Read the model definition and answer for the solid it produces. Units are mm, in the model's axes. Face numbers are marked on the shaded views. A direction names the side the tool comes from. Round coordinates to 2 decimals unless told otherwise and drop trailing zeros. Write each loop counter-clockwise with the first axis right and the second up, starting at its lowest first coordinate (ties: lowest second). Pieces come first, ordered by that corner, then holes. Notation, with made-up numbers: (8, 43) -> (13, 43) arc R6 cw to (13, 51) -> close; hole circle Ø8 at (30.5, 72). An arc over 180 degrees is marked (long way). Return JSON: item names as keys, results as strings. Group by question number.
(1) Given pin 1 (5.5 mm diameter, centred on x = 39, y = 5, fed in from -Z); pin 2 (8 mm diameter, centred on x = 39, y = 5, fed in from +Z); pin 3 (1.4 mm diameter, centred on x = 43.5, z = -7.5, fed in from -Y); pin 4 (2 mm diameter, centred on x = 26, y = -9.2, fed in from -Z), each flat-ended and moving along its own axis, determine where each tip first touches the part or whether it passes through.
(2) A cutting plane is placed at B-B on z = -11.25. Give the vertices of the cut face in (x, y).
(3) A cutting plane is placed at C-C on z = -8. Give the vertices of the cut face in (x, y), then the cut area to 3 significant figures.
(4) For the marked faces 4, 5 and 6, determine the directions among +Z, -Z, +X, -X, +Y, -Y from which every point of the face is accessible in a straight line to the end or side of a thin tool.
(5) A cutting plane is placed at A-A on x = 26. Give the vertices of the cut face in (y, z).
(6) Straight lines are drawn through the part: line 1 (X direction, y = 5, z = -11.05); line 2 (X direction, y = 6.25, z = -4.75); line 3 (Z direction, x = 29, y = 1.75). For each, find the intervals that lie inside material, in ascending order.
(7) A cutting plane is placed at D-D on x = 38.5. Give the vertices of the cut face in (y, z), then the cut area to 3 significant figures.
(8) The mould has two halves that part along X. Classify the marked faces 1, 2 and 3: released by +X, released by -X, zero draft, split by the parting line, or undercut.
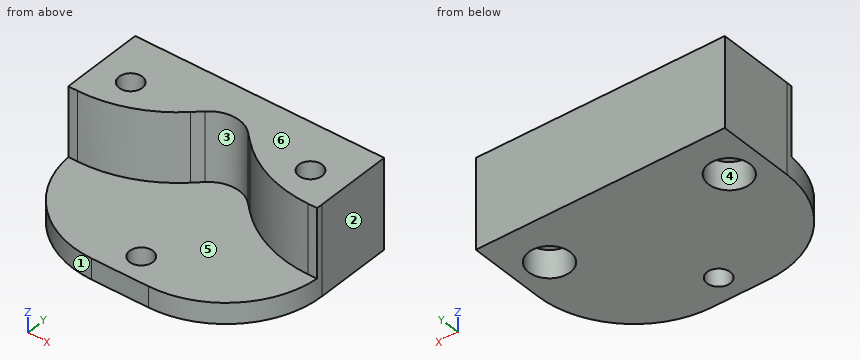
```python
from build123d import *

# Parameters (mm, degrees)
BOX001_W        = 36
BOX001_H        = 25
BOX001_DEPTH    = 13
SKETCH_R        = 1.68
POCKET005_DEPTH = 13.001
SKETCH014_W     = 13
SKETCH014_H     = 10
POCKET006_DEPTH = 36.001
SKETCH015_R     = 3
POCKET007_DEPTH = 4
POCKET008_DEPTH = 10
FILLET_R        = 18
FILLET001_R     = 4.5
FILLET002_R     = 13.9


with BuildPart() as part:
    # Box001 → Box001 (new body)
    with BuildSketch(Plane(origin=(8, -13, -13), x_dir=(1, 0, 0), z_dir=(0, 0, 1))):
        with Locations((18, 12.5)):
            Rectangle(BOX001_W, BOX001_H)
    extrude(amount=BOX001_DEPTH)

    # Sketch → Pocket005 (cut, through all)
    with BuildSketch(Plane(origin=(8, -13, -13), x_dir=(1, 0, 0), z_dir=(0, 0, -1))):
        with Locations((31, -18)):
            Circle(SKETCH_R)
        with Locations((5, -18)):
            Circle(SKETCH_R)
        with Locations((18, -3.8)):
            Circle(SKETCH_R)
    extrude(amount=-POCKET005_DEPTH, mode=Mode.SUBTRACT)

    # Sketch014 → Pocket006 (cut, through all)
    with BuildSketch(Plane(origin=(8, -13, -13), x_dir=(0, -1, 0), z_dir=(-1, 0, 0))):
        with Locations((-6.5, 8)):
            Rectangle(SKETCH014_W, SKETCH014_H)
    extrude(amount=-POCKET006_DEPTH, mode=Mode.SUBTRACT)

    # Sketch015 → Pocket007 (cut)
    with BuildSketch(Plane(origin=(8, -13, -13), x_dir=(1, 0, 0), z_dir=(0, 0, -1))):
        with Locations((5, -18)):
            Circle(SKETCH015_R)
        with Locations((31, -18)):
            Circle(SKETCH015_R)
    extrude(amount=-POCKET007_DEPTH, mode=Mode.SUBTRACT)

    # Sketch016 → Pocket008 (cut)
    with BuildSketch(Plane(origin=(8, -13, 0), x_dir=(1, 0, 0), z_dir=(0, 0, 1))):
        Polygon((8.5, 13), (18, 22), (27.5, 13), align=None)
    extrude(amount=-POCKET008_DEPTH, mode=Mode.SUBTRACT)

    # Fillet
    fillet_edges = [part.edges().sort_by_distance(p)[0] for p in [
        (16.5, 0, -5),
        (35.5, 0, -5),
    ]]
    fillet(fillet_edges, radius=FILLET_R)

    # Fillet001
    fillet001_edges = [part.edges().sort_by_distance(p)[0] for p in [
        (26, 9, -5),
    ]]
    fillet(fillet001_edges, radius=FILLET001_R)

    # Fillet002
    fillet002_edges = [part.edges().sort_by_distance(p)[0] for p in [
        (44, -13, -11.5),
        (8, -13, -11.5),
    ]]
    fillet(fillet002_edges, radius=FILLET002_R)


solid = part.part
```
Checks:
{
 "1": {"pin 1": "stops at z = -9", "pin 2": "stops at z = 0", "pin 3": "stops at y = 0", "pin 4": "passes through"},
 "2": {"outline": "(8, 0.9) arc R13.9 ccw to (21.9, -13) -> (30.1, -13) arc R13.9 ccw to (44, 0.9) -> (44, 12) -> (8, 12) -> close; hole circle Ø6 at (13, 5); hole circle Ø3.36 at (26, -9.2); hole circle Ø6 at (39, 5)"},
 "3": {"outline": "(8, 0.9) arc R13.9 ccw to (8.03, 0) -> (9.33, 0) arc R18 ccw to (21.71, 4.93) -> (22.91, 6.07) arc R4.5 cw to (29.09, 6.07) -> (30.29, 4.93) arc R18 ccw to (42.67, 0) -> (43.97, 0) arc R13.9 ccw to (44, 0.9) -> (44, 12) -> (8, 12) -> close; hole circle Ø3.36 at (13, 5); hole circle Ø3.36 at (39, 5)", "area": "320 mm^2"},
 "4": {"face 4": "-Z", "face 5": "+Z, -Y", "face 6": "+Z, +X, -X, +Y, -Y"},
 "5": {"outline": "(-13, -13) -> (-10.88, -13) -> (-10.88, -10) -> (-13, -10) -> close; (-7.52, -13) -> (12, -13) -> (12, 0) -> (7.3, 0) -> (7.3, -10) -> (-7.52, -10) -> close"},
 "6": {"line 1": "x = 8 to 10, 16 to 36, 42 to 44", "line 2": "x = 8 to 11.88, 14.12 to 23.11, 28.89 to 37.88, 40.12 to 44", "line 3": "z = -13 to -10"},
 "7": {"outline": "(-10.17, -13) -> (2.04, -13) -> (2.04, -9) -> (3.4, -9) -> (3.4, 0) -> (0.49, 0) -> (0.49, -10) -> (-10.17, -10) -> close; (6.6, -9) -> (7.96, -9) -> (7.96, -13) -> (12, -13) -> (12, 0) -> (6.6, 0) -> close", "area": "129 mm^2"},
 "8": {"face 1": "released by -X", "face 2": "released by +X", "face 3": "undercut"}
}
